from build123d import *

# Parameters (mm, degrees)
F0_W     = 76.2
F0_H     = 2133.6
F1_DEPTH = 4.7625
F2_R     = 24.13
F2_R_2   = 20.447
F3_DEPTH = 101.6
F5_DEPTH = 35.814


with BuildPart() as f1:
    # F0 (on Top) → F1 (new body)
    with BuildSketch(Plane.XY):
        with Locations((375.958569, -213.009804)):
            Rectangle(F0_W, F0_H)
    extrude(amount=-F1_DEPTH)

    # F2 (on face) → F3 (join)
    with BuildSketch(Plane.XY):
        with Locations((375.958569, 815.690196)):
            Circle(F2_R)
        with Locations((375.958569, 815.690196)):
            Circle(F2_R_2, mode=Mode.SUBTRACT)
    extrude(amount=-F3_DEPTH)

    # F4 (on face) → F5 (cut)
    with BuildSketch(Plane(origin=(0, 0, -4.7625), x_dir=(1, 0, 0), z_dir=(0, 0, -1))):
        Polygon((337.858569, 1107.854731), (414.058569, 1279.809804), (337.858569, 1279.809804), align=None)
    extrude(amount=-F5_DEPTH, mode=Mode.SUBTRACT)


solid = f1.part
Work out the finished part from the listing and answer in its coordinate system (mm). A direction names the side the tool comes from. Give positions to 0.01 mm unless a question says otherwise; leave off trailing zeros. Loops run counter-clockwise (first coordinate to the right, second up) from the corner with the lowest first, then second, coordinate; pieces in that order, holes last. Notation, with made-up numbers: (55.25, -4) - (68.25, -4) arc R16 cw to (68.25, 5) - close; hole circle Ø6 at (39.5, 4.5). An arc over 180 degrees is marked (long way). Answer in a Markdown table with one row per item.
(1) Section A-A (y = -245) is taken. Give the vertices of the cut face in (x, z).
Results list:
| item | result |
|---|---|
| outline | (337.86, -4.76) - (414.06, -4.76) - (414.06, 0) - (337.86, 0) - close |
(2) Consider L1, parallel to Y at x = 383, z = -95; L2, parallel to Y at x = 388, z = -42; L3, parallel to Z at x = 396, y = 80.5. Determine where each line is inside the solid, lowest interval first. Write a range as [from, to].
Results list:
| item | result |
|---|---|
| L1 | y = [792.61, 796.49], [834.89, 838.77] |
| L2 | y = [794.78, 799.16], [832.22, 836.6] |
| L3 | z = [-4.76, 0] |
(3) Flat-ended cylindrical pins translate along their axes: pin 1 Ø10 at (x, z) = (384.5, -48) entering from +Y; pin 2 Ø20.5 at (x, y) = (380.5, 807.5) entering from -Z; pin 3 Ø2 at (x, z) = (394, -67.5) entering from -Y. Find the tip coordinate at first contact, or state that the pin passes through.
Results list:
| item | result |
|---|---|
| pin 1 | stops at y = 839.56 |
| pin 2 | stops at z = -4.76 |
| pin 3 | stops at y = 798.61 |
(4) A tool of negligible diameter and unlimited length cuts with its end or side. For faces 4 (the face through (360.89, 829.51, -52.5)), 5 (the face through (375, -198, 0)), from which of +Z, -Z, +X, -X, +Y, -Y can it reach the whole face along a straight path? Write none if from no direction.
Results list:
| item | result |
|---|---|
| face 4 | -Z |
| face 5 | +Z, +X, -X, +Y, -Y |
(5) Section C-C (z = -31) is taken. Give the vertices of the cut face in (x, y).
Results list:
| item | result |
|---|---|
| outline | circle Ø48.26 at (375.96, 815.69); hole circle Ø40.89 at (375.96, 815.69) |
(6) For a pull along Y with two mould halves and no side action, classify faces 1 (the face through (387.09, 794.28, -52.5)), 2 (the face through (375.425, -1192.629, -2.415)), 3 (the face through (376, 816, -4.762)) as pulls with the +Y half, pulls with the -Y half, needs draft (parallel to the pull), parting line crosses it, or undercut.
Results list:
| item | result |
|---|---|
| face 1 | parting line crosses it |
| face 2 | pulls with the -Y half |
| face 3 | undercut |
(7) Section B-B (x = 373.5) is taken. Give the vertices of the cut face in (y, z).
Results list:
| item | result |
|---|---|
| outline | (-1188.28, -4.76) - (791.69, -4.76) - (791.69, -101.6) - (795.39, -101.6) - (795.39, -4.76) - (835.99, -4.76) - (835.99, -101.6) - (839.69, -101.6) - (839.69, -4.76) - (853.79, -4.76) - (853.79, 0) - (-1188.28, 0) - close |
